Check sheet for the modelled part. Datum: model origin and axes. Units: mm. Face numbers are marked on the shaded views. Round coordinates to 2 decimals unless told otherwise and drop trailing zeros. Write each loop counter-clockwise with the first axis right and the second up, starting at its lowest first coordinate (ties: lowest second). Pieces come first, ordered by that corner, then holes. Notation, with made-up numbers: (38, -10.5) - (86, -10.5) arc R18 cw to (86, 23.5) - close; hole circle Ø6 at (-17.75, -1.75). An arc over 180 degrees is marked (long way). Use one line per item in the form item = value. Start each with the question number.
1) Section check B-B (z = 50). Record the boundary of the cut face in (x, y).
2) Section check A-A (y = 64). Record the boundary of the cut face in (x, z).
3) Gauge pin test, flat ends, axial feed: P1, Ø3, axis at y = 66.5, z = 51.5, coming from the +X side; P2, Ø3, axis at y = 64, z = 9.5, coming from the +X side; P3, Ø2.5, axis at y = 19.5, z = 28, coming from the +X side. Record the tip position at first contact, or that the pin passes through.
4) Scan lines: probe 1 along Z at (x, y) = (11.8, 42); probe 2 along Z at (x, y) = (14.75, 43.5); probe 3 along Y at (x, z) = (11.25, 25.5). Record each from-to range of solid material in increasing order.
5) Section check D-D (y = 20). Record the boundary of the cut face in (x, z).
6) Section check C-C (z = 27). Record the boundary of the cut face in (x, y).
7) Draft check along Y on the marked faces 1, 2, 3 and 4. Enter one of: +Y half, -Y half, draft (parallel to the pull), parting line (faces both ways), or undercut.
from build123d import *

# Parameters (mm, degrees)
SKETCH_W        = 15.5
SKETCH_H        = 75
PAD_DEPTH       = 65
SKETCH001_R     = 3.25
POCKET_DEPTH    = 17
SKETCH002_R     = 2.6
POCKET001_DEPTH = 5.05
SKETCH003_R     = 5.35
POCKET002_DEPTH = 6.5


with BuildPart() as part:
    # Sketch → Pad (new body)
    with BuildSketch(Plane.XY):
        with Locations((7.75, 37.5)):
            Rectangle(SKETCH_W, SKETCH_H)
    extrude(amount=PAD_DEPTH)

    # Sketch001 (on Face2 of Pad) → Pocket (cut)
    with BuildSketch(Plane.YZ.offset(15.5)):
        with Locations((64, 50)):
            Circle(SKETCH001_R)
        with Locations((64, 10)):
            Circle(SKETCH001_R)
    extrude(amount=-POCKET_DEPTH, mode=Mode.SUBTRACT)

    # Sketch002 (on Face3 of Pocket) → Pocket001 (cut)
    with BuildSketch(Plane.YZ.offset(15.5)):
        with Locations((20, 45)):
            Circle(SKETCH002_R)
        with Locations((42, 45)):
            Circle(SKETCH002_R)
        with Locations((20, 27)):
            Circle(SKETCH002_R)
        with Locations((42, 27)):
            Circle(SKETCH002_R)
    extrude(amount=-POCKET001_DEPTH, mode=Mode.SUBTRACT)

    # Sketch003 (on Face3 of Pocket001) → Pocket002 (cut)
    with BuildSketch(Plane.YZ.offset(15.5)):
        with Locations((64, 50)):
            Circle(SKETCH003_R)
        with Locations((64, 10)):
            Circle(SKETCH003_R)
    extrude(amount=-POCKET002_DEPTH, mode=Mode.SUBTRACT)


solid = part.part
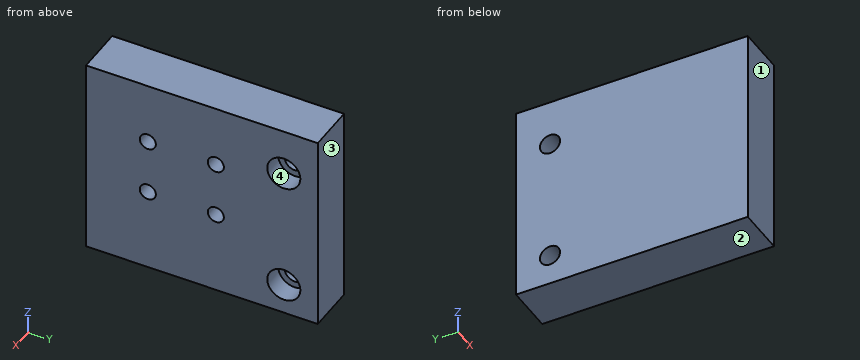
Results are:
q1.outline = (0, 0) - (15.5, 0) - (15.5, 58.65) - (9, 58.65) - (9, 60.75) - (0, 60.75) - close; (0, 67.25) - (9, 67.25) - (9, 69.35) - (15.5, 69.35) - (15.5, 75) - (0, 75) - close
q2.outline = (0, 0) - (15.5, 0) - (15.5, 4.65) - (9, 4.65) - (9, 6.75) - (0, 6.75) - close; (0, 13.25) - (9, 13.25) - (9, 15.35) - (15.5, 15.35) - (15.5, 44.65) - (9, 44.65) - (9, 46.75) - (0, 46.75) - close; (0, 53.25) - (9, 53.25) - (9, 55.35) - (15.5, 55.35) - (15.5, 65) - (0, 65) - close
q3.P1 = 9
q3.P2 = through
q3.P3 = 10.45
q4.probe_1 = 0 to 24.4, 29.6 to 42.4, 47.6 to 65
q4.probe_2 = 0 to 24.88, 29.12 to 42.88, 47.12 to 65
q4.probe_3 = 0 to 17.88, 22.12 to 39.88, 44.12 to 75
q5.outline = (0, 0) - (15.5, 0) - (15.5, 24.4) - (10.45, 24.4) - (10.45, 29.6) - (15.5, 29.6) - (15.5, 42.4) - (10.45, 42.4) - (10.45, 47.6) - (15.5, 47.6) - (15.5, 65) - (0, 65) - close
q6.outline = (0, 0) - (15.5, 0) - (15.5, 17.4) - (10.45, 17.4) - (10.45, 22.6) - (15.5, 22.6) - (15.5, 39.4) - (10.45, 39.4) - (10.45, 44.6) - (15.5, 44.6) - (15.5, 75) - (0, 75) - close
q7.face_1 = -Y half
q7.face_2 = draft
q7.face_3 = +Y half
q7.face_4 = undercut
